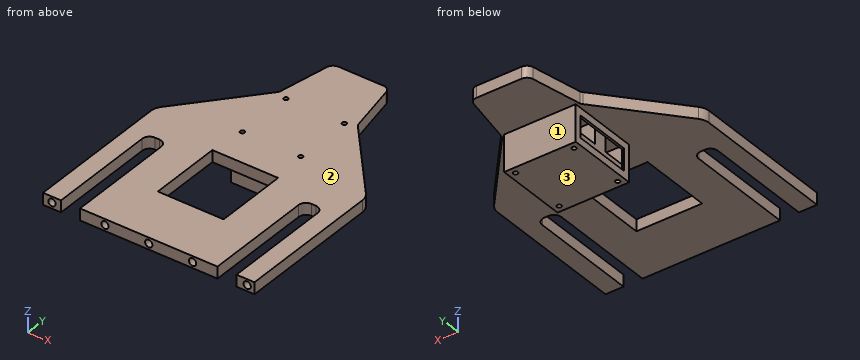
```python
from build123d import *

# Parameters (mm, degrees)
BOSS_EXTRUDE1_DEPTH    = 8
SKETCH2_W              = 45
SKETCH2_H              = 50
CUT_EXTRUDE1_DEPTH     = 342.206659287
SPLIT1_SURFACE_1_BACK  = 343.199
SPLIT1_SURFACE_1_DEPTH = 686.398
SPLIT1_SURFACE_2_BACK  = 343.199
SPLIT1_SURFACE_2_DEPTH = 686.398
SKETCH5_R              = 2.5
CUT_EXTRUDE6_DEPTH     = 5.2
SKETCH4_R              = 2.5
CUT_EXTRUDE7_DEPTH     = 5.2
SKETCH6_R              = 1.5
CUT_EXTRUDE8_DEPTH     = 342.206659287
SKETCH7_W              = 49
SKETCH7_H              = 49
SKETCH7_W_2            = 18
SKETCH7_H_2            = 18
BOSS_EXTRUDE2_DEPTH    = 15
SKETCH8_W              = 49
SKETCH8_H              = 49
SKETCH8_R              = 1.5
BOSS_EXTRUDE3_DEPTH    = 10
SKETCH9_W              = 15
SKETCH9_H              = 40
CUT_EXTRUDE9_DEPTH     = 1.5
SKETCH11_W             = 15
SKETCH11_H             = 40
CUT_EXTRUDE10_DEPTH    = 1.5


with BuildPart() as part:
    # Sketch1 → Boss-Extrude1 (new body)
    with BuildSketch(Plane.XY):
        with BuildLine():
            Line((70, 309.985818768), (85.299227191, 309.985818768))
            ThreePointArc((85.299227191, 309.985818768), (88.489017574, 308.836174247), (90.211957942, 305.915913694))
            Line((90.211957942, 305.915913694), (96.672728921, 271.790334282))
            ThreePointArc((96.672728921, 271.790334282), (97.06575438, 270.906904614), (97.621470019, 270.115641625))
            Line((97.621470019, 270.115641625), (139.950460317, 220.786053348))
            ThreePointArc((139.950460317, 220.786053348), (141.739336996, 217.746026552), (142.361429131, 214.274017901))
            Line((142.361429131, 214.274017901), (142.361429131, 30.859943174))
            ThreePointArc((142.361429131, 30.859943174), (140.896963037, 27.324409268), (137.361429131, 25.859943174))
            Line((137.361429131, 25.859943174), (114.717190871, 25.782318449))
            ThreePointArc((114.717190871, 25.782318449), (112.681998989, 25.341726514), (111.002773989, 24.110332733))
            Line((111.002773989, 24.110332733), (89.38285929, 0))
            Line((89.38285929, 0), (50.5, 0))
            Line((50.5, 0), (28.997226011, 24.110332733))
            ThreePointArc((28.997226011, 24.110332733), (27.318001011, 25.341726514), (25.282809129, 25.782318449))
            Line((25.282809129, 25.782318449), (2.638570869, 25.859943174))
            ThreePointArc((2.638570869, 25.859943174), (-0.896963037, 27.324409268), (-2.361429131, 30.859943174))
            Line((-2.361429131, 30.859943174), (-2.361429131, 214.274017901))
            ThreePointArc((-2.361429131, 214.274017901), (-1.739336996, 217.746026552), (0.049539683, 220.786053348))
            Line((0.049539683, 220.786053348), (42.261389271, 270.115641625))
            ThreePointArc((42.261389271, 270.115641625), (42.81710491, 270.906904614), (43.210130369, 271.790334282))
            Line((43.210130369, 271.790334282), (49.724618218, 305.923183314))
            ThreePointArc((49.724618218, 305.923183314), (51.449026762, 308.838533573), (54.635967087, 309.985818768))
            Line((54.635967087, 309.985818768), (70, 309.985818768))
        make_face()
        with BuildLine():
            Line((15.218798766, 54.807228462), (17.702103505, 54.807228462))
            ThreePointArc((17.702103505, 54.807228462), (21.420312934, 56.347361236), (22.960445707, 60.065570665))
            Line((22.960445707, 60.065570665), (22.960445707, 189.807228462))
            ThreePointArc((22.960445707, 189.807228462), (21.495979613, 193.342762368), (17.960445707, 194.807228462))
            Line((17.960445707, 194.807228462), (14.960456564, 194.807228462))
            ThreePointArc((14.960456564, 194.807228462), (11.424922658, 193.342762368), (9.960456564, 189.807228462))
            Line((9.960456564, 189.807228462), (9.960456564, 60.065570665))
            ThreePointArc((9.960456564, 60.065570665), (11.500589337, 56.347361236), (15.218798766, 54.807228462))
        make_face(mode=Mode.SUBTRACT)
        with BuildLine():
            Line((125.039543436, 54.807228462), (122.039554293, 54.807228462))
            ThreePointArc((122.039554293, 54.807228462), (118.504020387, 56.271694556), (117.039554293, 59.807228462))
            Line((117.039554293, 59.807228462), (117.039554293, 189.807228462))
            ThreePointArc((117.039554293, 189.807228462), (118.504020387, 193.342762368), (122.039554293, 194.807228462))
            Line((122.039554293, 194.807228462), (125.039543436, 194.807228462))
            ThreePointArc((125.039543436, 194.807228462), (128.575077342, 193.342762368), (130.039543436, 189.807228462))
            Line((130.039543436, 189.807228462), (130.039543436, 59.807228462))
            ThreePointArc((130.039543436, 59.807228462), (128.575077342, 56.271694556), (125.039543436, 54.807228462))
        make_face(mode=Mode.SUBTRACT)
    extrude(amount=BOSS_EXTRUDE1_DEPTH)

    # Sketch2 → Cut-Extrude1 (cut, through all)
    with BuildSketch(Plane.XY.offset(8)):
        with Locations((69.88285929, 179.008918923)):
            Rectangle(SKETCH2_W, SKETCH2_H)
    extrude(amount=-CUT_EXTRUDE1_DEPTH, mode=Mode.SUBTRACT)


with BuildPart() as body_2:
    # Split1: the piece behind the surface
    add(part.part)
    # Split1 surface: a surface, the sketch's curves swept straight by 686.398 mm
    with BuildLine(Plane(origin=(0, 0, 0), x_dir=(-1, 0, 0), z_dir=(0, 0, -1)).offset(-SPLIT1_SURFACE_1_BACK), mode=Mode.PRIVATE) as split1_surface_1_path:
        Line((-142.361429131, 115.359943174), (2.361429131, 115.359943174))
    split1_surface_1 = Shell.extrude(split1_surface_1_path.wire(), (0 * SPLIT1_SURFACE_1_DEPTH, 0 * SPLIT1_SURFACE_1_DEPTH, -1 * SPLIT1_SURFACE_1_DEPTH))
    split(bisect_by=split1_surface_1, keep=Keep.BOTTOM)

    # Sketch5 → Cut-Extrude6 (cut)
    with BuildSketch(Plane(origin=(0, 115.359943174, -115.359943174), x_dir=(1, 0, 0), z_dir=(0, -1, 0))):
        with Locations(Location((70, 119.359943174, 0), (0, 0, 270))):
            Circle(SKETCH5_R)
        with Locations(Location((40, 119.359943174, 0), (0, 0, 270))):
            Circle(SKETCH5_R)
        with Locations(Location((2.638570869, 119.359943174, 0), (0, 0, 270))):
            Circle(SKETCH5_R)
    extrude(amount=CUT_EXTRUDE6_DEPTH, mode=Mode.SUBTRACT)


with BuildPart() as part_1:
    add(part.part)

    # Split1: split by a surface, the side it looks to stays
    # Split1 surface: a surface, the sketch's curves swept straight by 686.398 mm
    with BuildLine(Plane(origin=(0, 0, 0), x_dir=(-1, 0, 0), z_dir=(0, 0, -1)).offset(-SPLIT1_SURFACE_2_BACK), mode=Mode.PRIVATE) as split1_surface_2_path:
        Line((-142.361429131, 115.359943174), (2.361429131, 115.359943174))
    split1_surface_2 = Shell.extrude(split1_surface_2_path.wire(), (0 * SPLIT1_SURFACE_2_DEPTH, 0 * SPLIT1_SURFACE_2_DEPTH, -1 * SPLIT1_SURFACE_2_DEPTH))
    split(bisect_by=split1_surface_2, keep=Keep.TOP)

    # Sketch4 → Cut-Extrude7 (cut)
    with BuildSketch(Plane(origin=(0, 115.359943174, 0), x_dir=(-1, 0, 0), z_dir=(0, -1, 0))):
        with Locations(Location((-70, -4, 0), (0, 0, 270))):
            Circle(SKETCH4_R)
        with Locations(Location((-40, -4, 0), (0, 0, 270))):
            Circle(SKETCH4_R)
        with Locations(Location((-100, -4, 0), (0, 0, 270))):
            Circle(SKETCH4_R)
        with Locations(Location((-137.361429131, -4, 0), (0, 0, 90))):
            Circle(SKETCH4_R)
        with Locations(Location((-3.799513716, -4, 0), (0, 0, 270))):
            Circle(SKETCH4_R)
    extrude(amount=-CUT_EXTRUDE7_DEPTH, mode=Mode.SUBTRACT)

    # Sketch6 → Cut-Extrude8 (cut, through all)
    with BuildSketch(Plane.XY.offset(8)):
        with Locations((50.000130369, 267.980334282)):
            Circle(SKETCH6_R)
        with Locations((90.000130369, 267.980334282)):
            Circle(SKETCH6_R)
        with Locations((90.000130369, 227.980334282)):
            Circle(SKETCH6_R)
        with Locations((50.000130369, 227.980334282)):
            Circle(SKETCH6_R)
    extrude(amount=-CUT_EXTRUDE8_DEPTH, mode=Mode.SUBTRACT)

    # Sketch7 → Boss-Extrude2 (add)
    with BuildSketch(Plane(origin=(0, 0, 0), x_dir=(-1, 0, 0), z_dir=(0, 0, -1))):
        with Locations((-70.000130369, 247.980334282)):
            Rectangle(SKETCH7_W, SKETCH7_H)
        with Locations((-56.000130369, 261.980334282)):
            Rectangle(SKETCH7_W_2, SKETCH7_H_2, mode=Mode.SUBTRACT)
        with Locations((-84.000130369, 261.980334282)):
            Rectangle(SKETCH7_W_2, SKETCH7_H_2, mode=Mode.SUBTRACT)
        with Locations((-84.000130369, 233.980334282)):
            Rectangle(SKETCH7_W_2, SKETCH7_H_2, mode=Mode.SUBTRACT)
        with Locations((-56.000130369, 233.980334282)):
            Rectangle(SKETCH7_W_2, SKETCH7_H_2, mode=Mode.SUBTRACT)
    extrude(amount=BOSS_EXTRUDE2_DEPTH)

    # Sketch8 → Boss-Extrude3 (add)
    with BuildSketch(Plane(origin=(0, 0, -15), x_dir=(-1, 0, 0), z_dir=(0, 0, -1))):
        with Locations((-70.000130369, 247.980334282)):
            Rectangle(SKETCH8_W, SKETCH8_H)
        with Locations(Location((-50.000130369, 267.980334282, 0), (0, 0, 180))):
            Circle(SKETCH8_R, mode=Mode.SUBTRACT)
        with Locations(Location((-90.000130369, 267.980334282, 0), (0, 0, 180))):
            Circle(SKETCH8_R, mode=Mode.SUBTRACT)
        with Locations(Location((-50.000130369, 227.980334282, 0), (0, 0, 180))):
            Circle(SKETCH8_R, mode=Mode.SUBTRACT)
        with Locations(Location((-90.000130369, 227.980334282, 0), (0, 0, 180))):
            Circle(SKETCH8_R, mode=Mode.SUBTRACT)
    extrude(amount=BOSS_EXTRUDE3_DEPTH)

    # Sketch9 → Cut-Extrude9 (cut)
    with BuildSketch(Plane.ZY.offset(-45.500130369)):
        with Locations((-12.5, 247.980334282)):
            Rectangle(SKETCH9_W, SKETCH9_H)
    extrude(amount=-CUT_EXTRUDE9_DEPTH, mode=Mode.SUBTRACT)

    # Sketch11 → Cut-Extrude10 (cut)
    with BuildSketch(Plane(origin=(94.500130369, 0, 0), x_dir=(0, 0, -1), z_dir=(1, 0, 0))):
        with Locations((12.5, 247.980334282)):
            Rectangle(SKETCH11_W, SKETCH11_H)
    extrude(amount=-CUT_EXTRUDE10_DEPTH, mode=Mode.SUBTRACT)


solid = part_1.part
```
Geometry: final body of the model. Coordinates: model frame, mm. Face numbers are marked on the shaded views. Round coordinates to 2 decimals unless told otherwise and drop trailing zeros. Order: outer loops, then holes, each group sorted by start corner. A loop starts at its lowest first (then second) coordinate and runs counter-clockwise, first axis right, second up. Notation, with made-up numbers: (53.5, -12.5) - (102.5, -12.5) arc R15 ccw to (102.5, -7.5) - close; hole circle Ø5 at (7.5, 36.25). An arc over 180 degrees is marked (long way). Write item = value, one per line. Start each with the question number.
Q1. Cut plane B-B on z = -22. Return the cut outline in (x, y).
Q2. Cut plane D-D on z = -13. Return the cut outline in (x, y), and give its area (3 significant figures).
Q3. Ray query, line 1 (X direction, y = 137, z = 6); line 2 (Y direction, x = 63, z = -12); line 3 (Z direction, x = 92.5, y = 267). Return the intervals inside material, ascending. Write a range as from..to.
Q4. Pull-direction query (Z, two-part tool) for the marked faces 1, 2 and 3; classes: +Z half, -Z half, draft (parallel to the pull), parting line (faces both ways), or undercut.
Q5. Cut plane A-A on x = 70. Return the cut outline in (y, z).
Q6. Pin query (flat end, axial travel): pin 1 (8 mm diameter, centred on y = 222.5, z = -5, fed in from -X); pin 2 (1.8 mm diameter, centred on x = 50, y = 227.98, fed in from -Z); pin 3 (3 mm diameter, centred on y = 251, z = -10, fed in from +X); pin 4 (4.5 mm diameter, centred on x = 3.8, z = 4, fed in from +Y). Return the tip coordinate at first contact, or that it passes through.
Q7. Cut plane C-C on y = 157.5. Return the cut outline in (x, z), and give its area (3 significant figures).
Outcome:
q1.outline = (45.5, 223.48) - (94.5, 223.48) - (94.5, 272.48) - (45.5, 272.48) - close; hole circle Ø3 at (50, 227.98); hole circle Ø3 at (50, 267.98); hole circle Ø3 at (90, 227.98); hole circle Ø3 at (90, 267.98)
q2.outline = (45.5, 223.48) - (94.5, 223.48) - (94.5, 227.98) - (93, 227.98) - (93, 224.98) - (75, 224.98) - (75, 242.98) - (93, 242.98) - (93, 252.98) - (75, 252.98) - (75, 270.98) - (93, 270.98) - (93, 267.98) - (94.5, 267.98) - (94.5, 272.48) - (45.5, 272.48) - (45.5, 267.98) - (47, 267.98) - (47, 270.98) - (65, 270.98) - (65, 252.98) - (47, 252.98) - (47, 242.98) - (65, 242.98) - (65, 224.98) - (47, 224.98) - (47, 227.98) - (45.5, 227.98) - close
q2.area = 985 mm^2
q3.line_1 = -2.36..9.96, 22.96..117.04, 130.04..142.36
q3.line_2 = 223.48..224.98, 242.98..252.98, 270.98..272.48
q3.line_3 = -25..-15, 0..8
q4.face_1 = draft
q4.face_2 = +Z half
q4.face_3 = -Z half
q5.outline = (115.36, 0) - (154.01, 0) - (154.01, 8) - (115.36, 8) - (115.36, 6.5) - (120.56, 6.5) - (120.56, 1.5) - (115.36, 1.5) - close; (204.01, 0) - (223.48, 0) - (223.48, -25) - (272.48, -25) - (272.48, 0) - (309.99, 0) - (309.99, 8) - (204.01, 8) - close
q6.pin_1 = 45.5
q6.pin_2 = through
q6.pin_3 = 93
q6.pin_4 = 227.8
q7.outline = (-2.36, 0) - (9.96, 0) - (9.96, 8) - (-2.36, 8) - close; (22.96, 0) - (47.38, 0) - (47.38, 8) - (22.96, 8) - close; (92.38, 0) - (117.04, 0) - (117.04, 8) - (92.38, 8) - close; (130.04, 0) - (142.36, 0) - (142.36, 8) - (130.04, 8) - close
q7.area = 590 mm^2
